Read the model definition and answer for the solid it produces. Units are mm, in the model's axes. A direction names the side the tool comes from. Give positions to 0.01 mm unless a question says otherwise; leave off trailing zeros. Order: outer loops, then holes, each group sorted by start corner. A loop starts at its lowest first (then second) coordinate and runs counter-clockwise, first axis right, second up.
Item 1: Find the intervals of material crossed by line 1 along Y through (x, z) = (133.5, 7.5); line 2 along Y through (x, z) = (185, 13.5); line 3 along Z through (x, y) = (46.5, 66.5), in increasing order.
Item 2: Which of the six approach directions +Z, -Z, +X, -X, +Y, -Y give full straight-line access (tool end or side, diameter ignored) to faces 4 (the face through (99, -2.073, 5)), 5 (the face through (99, -1.473, 5)), 6 (the face through (99, 0.6, 16)), 7 (the face through (99, 0, 16)), 8 (the face through (99, 96.627, 144))?
Item 3: A cutting plane is placed at C-C (z = 108.5). Write down the section's boundary in (x, y).
Item 4: A cutting plane is placed at B-B (x = 118). Write down the section's boundary in (y, z), plus the area to 3 significant figures.
Item 5: Given pin 1 Ø8 at (x, y) = (144, 79) entering from +Z; pin 2 Ø2.5 at (x, z) = (201, 13.5) entering from -Y; pin 3 Ø21.5 at (y, z) = (56, 15) entering from -X, each flat-ended and moving along its own axis, determine where each tip first touches the part or whether it passes through.
Item 6: A cutting plane is placed at A-A (y = 59). Write down the section's boundary in (x, z), plus the area to 3 significant figures.
Item 7: The mould has two halves that part along Z. Classify faces 1 (the face through (99, 47, -0.6)), 2 (the face through (201.737, 47, 11)), 3 (the face through (99, 97.327, 76)): +Z half, -Z half, draft (parallel to the pull), parting line (faces both ways), or undercut.
from build123d import *

# Parameters (mm, degrees)
SKETCH1_W                    = 100
SKETCH1_H                    = 200
BASE_FLANGE1_DEPTH           = 0.6
EDGE_FLANGE1_STRIP_W         = 3.8732
EDGE_FLANGE1_STRIP_H         = 0.6
EDGE_FLANGE1_STRIP_CUT_DEPTH = 200
EDGE_FLANGE1_DEPTH           = 200
HEM1_DEPTH                   = 200
HEM1_2_DEPTH                 = 200
EDGE_FLANGE2_STRIP_W         = 3.8732
EDGE_FLANGE2_STRIP_H         = 0.6
EDGE_FLANGE2_STRIP_CUT_DEPTH = 200
EDGE_FLANGE2_DEPTH           = 200
JOG2_DEPTH                   = 200
JOG2_2_DEPTH                 = 200
EDGE_FLANGE4_DEPTH           = 97.3268


# Read off the part's stored shape, not the designer's step: Hem1, Jog2
# Sheet-metal steps are written as plain solids
with BuildPart() as part:
    # Sketch1 → Base-Flange1 (new body)
    with BuildSketch(Plane(origin=(0, 0, 0), x_dir=(0, 1, 0), z_dir=(0, 0, 1))):
        with Locations((50, -100)):
            Rectangle(SKETCH1_W, SKETCH1_H)
    extrude(amount=-BASE_FLANGE1_DEPTH)

    # Edge-Flange1 strip (across the edge) → Edge-Flange1 strip cut (cut)
    with BuildSketch(Plane(origin=(200, 100, 0), x_dir=(0, -1, 0), z_dir=(-1, 0, 0))):
        with Locations((-0.6, -0.3)):
            Rectangle(EDGE_FLANGE1_STRIP_W, EDGE_FLANGE1_STRIP_H)
    extrude(amount=EDGE_FLANGE1_STRIP_CUT_DEPTH, mode=Mode.SUBTRACT)

    # Edge-Flange1 section (across the edge) → Edge-Flange1 (add)
    with BuildSketch(Plane(origin=(200, 100, 0), x_dir=(0, -1, 0), z_dir=(-1, 0, 0))):
        with BuildLine():
            Line((0, 0.7366), (0, 149.4))
            Line((0, 149.4), (0.6, 149.4))
            Line((0.6, 149.4), (0.6, 0.7366))
            ThreePointArc((0.6, 0.7366), (0.815745145, 0.215745145), (1.3366, 0))
            Line((1.3366, 0), (1.3366, -0.6))
            ThreePointArc((1.3366, -0.6), (0.391481076, -0.208518924), (0, 0.7366))
        make_face()
    extrude(amount=EDGE_FLANGE1_DEPTH)

    # Hem1 outline → Hem1 (cut)
    with BuildSketch(Plane.YZ):
        with BuildLine():
            Line((99.4, 149.4), (99.4, 149.39807407))
            ThreePointArc((99.4, 149.39807407), (99.826969601, 149.191588043), (100, 148.75))
            Line((100, 148.75), (100, 149.4))
            Line((100, 149.4), (99.4, 149.4))
        make_face()
    extrude(amount=HEM1_DEPTH, mode=Mode.SUBTRACT)

    # Hem1 2 outline → Hem1 2 (add)
    with BuildSketch(Plane.YZ):
        with BuildLine():
            Line((98.7, 139.4), (99.3, 139.4))
            Line((99.3, 139.4), (99.3, 148.75))
            ThreePointArc((99.3, 148.75), (99.35, 148.8), (99.4, 148.75))
            Line((99.4, 148.75), (99.4, 149.39807407))
            ThreePointArc((99.4, 149.39807407), (98.908411957, 149.226969601), (98.7, 148.75))
            Line((98.7, 148.75), (98.7, 139.4))
        make_face()
    extrude(amount=HEM1_2_DEPTH)

    # Edge-Flange2 strip (across the edge) → Edge-Flange2 strip cut (cut)
    with BuildSketch(Plane.YZ):
        with Locations((-0.6, -0.3)):
            Rectangle(EDGE_FLANGE2_STRIP_W, EDGE_FLANGE2_STRIP_H)
    extrude(amount=EDGE_FLANGE2_STRIP_CUT_DEPTH, mode=Mode.SUBTRACT)

    # Edge-Flange2 section (across the edge) → Edge-Flange2 (add)
    with BuildSketch(Plane.YZ):
        with BuildLine():
            Line((0, 0.7366), (0, 20.4))
            Line((0, 20.4), (0.6, 20.4))
            Line((0.6, 20.4), (0.6, 0.7366))
            ThreePointArc((0.6, 0.7366), (0.815745145, 0.215745145), (1.3366, 0))
            Line((1.3366, 0), (1.3366, -0.6))
            ThreePointArc((1.3366, -0.6), (0.391481076, -0.208518924), (0, 0.7366))
        make_face()
    extrude(amount=EDGE_FLANGE2_DEPTH)

    # Jog2 outline → Jog2 (cut)
    with BuildSketch(Plane.YZ):
        with BuildLine():
            ThreePointArc((0.6, 11.382443736), (0.440480949, 10.74921392), (0, 10.26713212))
            Line((0, 10.26713212), (0, 0.7366))
            ThreePointArc((0, 0.7366), (0.056516982, 0.352039176), (0.221288384, 0))
            Line((0.221288384, 0), (1.3366, 0))
            ThreePointArc((1.3366, 0), (0.815745145, 0.215745145), (0.6, 0.7366))
            Line((0.6, 0.7366), (0.6, 11.382443736))
        make_face()
        with BuildLine():
            ThreePointArc((97.705511616, 0), (97.223429816, -0.440480949), (96.5902, -0.6))
            Line((96.5902, -0.6), (98.6634, -0.6))
            ThreePointArc((98.6634, -0.6), (99.608518924, -0.208518924), (100, 0.7366))
            Line((100, 0.7366), (100, 148.75))
            ThreePointArc((100, 148.75), (99.35, 149.4), (98.7, 148.75))
            Line((98.7, 148.75), (98.7, 139.4))
            Line((98.7, 139.4), (99.3, 139.4))
            Line((99.3, 139.4), (99.3, 148.75))
            ThreePointArc((99.3, 148.75), (99.35, 148.8), (99.4, 148.75))
            Line((99.4, 148.75), (99.4, 0.7366))
            ThreePointArc((99.4, 0.7366), (99.184254855, 0.215745145), (98.6634, 0))
            Line((98.6634, 0), (97.705511616, 0))
        make_face()
    extrude(amount=JOG2_DEPTH, mode=Mode.SUBTRACT)

    # Jog2 2 outline → Jog2 2 (add)
    with BuildSketch(Plane.YZ):
        with BuildLine():
            ThreePointArc((-0.7366, 10.645843736), (-1.681718924, 10.25436266), (-2.0732, 9.309243736))
            Line((-2.0732, 9.309243736), (-2.0732, 0.7366))
            ThreePointArc((-2.0732, 0.7366), (-1.681718924, -0.208518924), (-0.7366, -0.6))
            Line((-0.7366, -0.6), (1.3366, -0.6))
            ThreePointArc((1.3366, -0.6), (0.703370184, -0.440480949), (0.221288384, 0))
            Line((0.221288384, 0), (-0.7366, 0))
            ThreePointArc((-0.7366, 0), (-1.257454855, 0.215745145), (-1.4732, 0.7366))
            Line((-1.4732, 0.7366), (-1.4732, 9.309243736))
            ThreePointArc((-1.4732, 9.309243736), (-1.257454855, 9.830098591), (-0.7366, 10.045843736))
            ThreePointArc((-0.7366, 10.045843736), (-0.352039176, 10.102360718), (0, 10.26713212))
            Line((0, 10.26713212), (0, 11.382443736))
            ThreePointArc((0, 11.382443736), (-0.215745145, 10.861588881), (-0.7366, 10.645843736))
        make_face()
        with BuildLine():
            Line((96.5902, 0), (97.705511616, 0))
            ThreePointArc((97.705511616, 0), (97.870283018, 0.352039176), (97.9268, 0.7366))
            Line((97.9268, 0.7366), (97.9268, 148.75))
            ThreePointArc((97.9268, 148.75), (97.2768, 149.4), (96.6268, 148.75))
            Line((96.6268, 148.75), (96.6268, 139.4))
            Line((96.6268, 139.4), (97.2268, 139.4))
            Line((97.2268, 139.4), (97.2268, 148.75))
            ThreePointArc((97.2268, 148.75), (97.2768, 148.8), (97.3268, 148.75))
            Line((97.3268, 148.75), (97.3268, 0.7366))
            ThreePointArc((97.3268, 0.7366), (97.111054855, 0.215745145), (96.5902, 0))
        make_face()
    extrude(amount=JOG2_2_DEPTH)

    # Edge-Flange4 section (across the edge) → Edge-Flange4 (add)
    with BuildSketch(Plane(origin=(201.7366, -0.7366, 0), x_dir=(-1, 0, 0), z_dir=(0, 1, 0))):
        with BuildLine():
            Line((-0.6, 0.7366), (-0.6, 20.4))
            Line((-0.6, 20.4), (0, 20.4))
            Line((0, 20.4), (0, 0.7366))
            ThreePointArc((0, 0.7366), (0.215745145, 0.215745145), (0.7366, 0))
            Line((0.7366, 0), (1.7366, 0))
            Line((1.7366, 0), (1.7366, -0.6))
            Line((1.7366, -0.6), (0.7366, -0.6))
            ThreePointArc((0.7366, -0.6), (-0.208518924, -0.208518924), (-0.6, 0.7366))
        make_face()
    extrude(amount=EDGE_FLANGE4_DEPTH)


solid = part.part
Response values:
1. line 1: y = -2.07 to -1.47, 97.33 to 97.93
1. line 2: y = 0 to 0.6, 97.33 to 97.93
1. line 3: z = -0.6 to 0
2. face 4: +Z, -Z, +X, -X, -Y
2. face 5: +X, -X
2. face 6: +Z, -X
2. face 7: +Z, -X, -Y
2. face 8: +Z, +X, -X, -Y
3. outline: (0, 97.33) - (200, 97.33) - (200, 97.93) - (0, 97.93) - close
4. outline: (-2.07, 0.74) arc R1.34 ccw to (-0.74, -0.6) - (96.59, -0.6) arc R1.34 ccw to (97.93, 0.74) - (97.93, 148.75) arc R0.65 ccw to (96.63, 148.75) - (96.63, 139.4) - (97.23, 139.4) - (97.23, 148.75) arc R0.05 cw to (97.33, 148.75) - (97.33, 0.74) arc R0.74 cw to (96.59, 0) - (-0.74, 0) arc R0.74 cw to (-1.47, 0.74) - (-1.47, 9.31) arc R0.74 cw to (-0.74, 10.05) arc R1.34 ccw to (0.6, 11.38) - (0.6, 20.4) - (0, 20.4) - (0, 11.38) arc R0.74 cw to (-0.74, 10.65) arc R1.34 ccw to (-2.07, 9.31) - close
4. area: 168 mm2
5. pin 1: stops at z = 0
5. pin 2: stops at y = -0.74
5. pin 3: stops at x = 201.74
6. outline: (0, -0.6) - (201, -0.6) arc R1.34 ccw to (202.34, 0.74) - (202.34, 20.4) - (201.74, 20.4) - (201.74, 0.74) arc R0.74 cw to (201, 0) - (0, 0) - close
6. area: 133 mm2
7. face 1: -Z half
7. face 2: draft
7. face 3: undercut
